```python
from build123d import *

# Parameters (mm, degrees)
SKETCH_1_R      = 4.55
SKETCH_1_R_2    = 2.8
EXTRUDE_1_DEPTH = 2.9
SKETCH_2_W      = 10
SKETCH_2_H      = 10
SKETCH_2_R      = 1.55
EXTRUDE_2_DEPTH = 1.4
SKETCH_3_W      = 1.25
SKETCH_3_H      = 10
EXTRUDE_3_DEPTH = 2.1


with BuildPart() as part:
    # Эскиз1 → Вытянуть1 (new body)
    with BuildSketch(Plane.XY):
        Circle(SKETCH_1_R)
        Circle(SKETCH_1_R_2, mode=Mode.SUBTRACT)
    extrude(amount=EXTRUDE_1_DEPTH)

    # Эскиз2 → Вытянуть2 (add)
    with BuildSketch(Plane.XY.offset(2.9)):
        Rectangle(SKETCH_2_W, SKETCH_2_H)
        Circle(SKETCH_2_R, mode=Mode.SUBTRACT)
    extrude(amount=EXTRUDE_2_DEPTH)

    # Эскиз3 → Вытянуть3 (add)
    with BuildSketch(Plane.XY.offset(4.3)):
        with Locations((-4.375, 0)):
            Rectangle(SKETCH_3_W, SKETCH_3_H)
        with Locations((4.375, 0)):
            Rectangle(SKETCH_3_W, SKETCH_3_H)
    extrude(amount=EXTRUDE_3_DEPTH)


solid = part.part
```
Model file for the job. Use its own axes, mm. A direction names the side the tool comes from. Coordinates: 2 decimals unless noted, no trailing zeros. Write each loop counter-clockwise with the first axis right and the second up, starting at its lowest first coordinate (ties: lowest second). Pieces come first, ordered by that corner, then holes. Notation, with made-up numbers: (-23.75, 31.25) - (31.25, 31.25) arc R16 ccw to (31.25, 39.25) - close; hole circle Ø8 at (-2.75, 10.25). An arc over 180 degrees is marked (long way). One line per question, with ' | ' between items. Start each with the question number.
Q1. Cut at C-C, the plane y = 1. List the corners of the cut face in (x, z).
Q2. Cut at A-A, the plane x = 0. List the corners of the cut face in (y, z), then the cut area to 3 significant figures.
Q3. Pin check, flat tips, straight feed: pin 1 (1.5 mm diameter, centred on y = -3, z = 2, fed in from -X); pin 2 (2 mm diameter, centred on x = 1.5, y = 2, fed in from +Z); pin 3 (1.5 mm diameter, centred on x = -3.5, y = 3, fed in from -Z); pin 4 (3.5 mm diameter, centred on x = 0, y = 0, fed in from -Z). Stop position of each tip, or through.
Q4. Cut at B-B, the plane z = 5.5. List the corners of the cut face in (x, y), then the cut area to 3 significant figures.
Q5. Cut at D-D, the plane z = 0.5. List the corners of the cut face in (x, y).
Q6. 3-axis set-ups, long thin cutter, end or side, ignore diameter. For faces 4 (the face through (-4, 0, 6.4)), 5 (the face through (-0.99, -4.44, 1.43)), 6 (the face through (-2, 0, 4.3)): which of +Z, -Z, +X, -X, +Y, -Y reach the whole face in a straight line?
Q7. Pull direction Y, two halves, no side cores. Call faces 1 (the face through (0, 5, 4)), 2 (the face through (1.21, -1.21, 2.9)), 3 (the face through (3.75, 0, 5)): pulls with the +Y half, pulls with the -Y half, needs draft (parallel to the pull), parting line crosses it, or undercut.
Q8. Drill centre lines: line 1 (Y direction, x = 0, z = 0.85); line 2 (X direction, y = -0.75, z = 5); line 3 (Z direction, x = -4, y = 3.25). Where is each one in solid material? Low to high. Write a range as [from, to].
Answer below:
1) outline: (-5, 2.9) - (-4.44, 2.9) - (-4.44, 0) - (-2.62, 0) - (-2.62, 2.9) - (-1.18, 2.9) - (-1.18, 4.3) - (-3.75, 4.3) - (-3.75, 6.4) - (-5, 6.4) - close; (1.18, 2.9) - (2.62, 2.9) - (2.62, 0) - (4.44, 0) - (4.44, 2.9) - (5, 2.9) - (5, 6.4) - (3.75, 6.4) - (3.75, 4.3) - (1.18, 4.3) - close
2) outline: (-5, 2.9) - (-4.55, 2.9) - (-4.55, 0) - (-2.8, 0) - (-2.8, 2.9) - (-1.55, 2.9) - (-1.55, 4.3) - (-5, 4.3) - close; (1.55, 2.9) - (2.8, 2.9) - (2.8, 0) - (4.55, 0) - (4.55, 2.9) - (5, 2.9) - (5, 4.3) - (1.55, 4.3) - close | area: 19.8 mm^2
3) pin 1: x = -3.95 | pin 2: z = 4.3 | pin 3: z = 0 | pin 4: z = 2.9
4) outline: (-5, -5) - (-3.75, -5) - (-3.75, 5) - (-5, 5) - close; (3.75, -5) - (5, -5) - (5, 5) - (3.75, 5) - close | area: 25.0 mm^2
5) outline: circle Ø9.1 at (0, 0); hole circle Ø5.6 at (0, 0)
6) face 4: +Z, +X, -X, +Y, -Y | face 5: -Z | face 6: +Z, +Y, -Y
7) face 1: pulls with the +Y half | face 2: undercut | face 3: needs draft
8) line 1: [-4.55, -2.8], [2.8, 4.55] | line 2: [-5, -3.75], [3.75, 5] | line 3: [2.9, 6.4]
